Read the model definition and answer for the solid it produces. Units are mm, in the model's axes. A direction names the side the tool comes from. Give positions to 0.01 mm unless a question says otherwise; leave off trailing zeros. Write each loop counter-clockwise with the first axis right and the second up, starting at its lowest first coordinate (ties: lowest second). Pieces come first, ordered by that corner, then holes. Notation, with made-up numbers: (49.5, -16.5) -> (69.5, -16.5) arc R19 ccw to (69.5, -7.5) -> close; hole circle Ø11 at (26, -3.5). An arc over 180 degrees is marked (long way). Write item = value, one per line.
from build123d import *

# Parameters (mm, degrees)
F0_R          = 9.5
F1_DEPTH      = 42
F1_DEPTH_BACK = 59
F2_R          = 16
F3_DEPTH      = 2.5
F3_DEPTH_BACK = 2.5
F4_R          = 4


with BuildPart() as f1:
    # F0 (on Top) → F1 (new body, two sides)
    with BuildSketch(Plane.XY) as f1_sk:
        Circle(F0_R)
    extrude(amount=F1_DEPTH)
    extrude(f1_sk.sketch, amount=-F1_DEPTH_BACK)

    # F2 (on Top) → F3 (join, two sides)
    with BuildSketch(Plane.XY) as f3_sk:
        Circle(F2_R)
    extrude(amount=F3_DEPTH)
    extrude(f3_sk.sketch, amount=-F3_DEPTH_BACK)

    # F4
    f4_edges = [f1.edges().sort_by_distance(p)[0] for p in [
        (-9.5, 0, -2.5),
        (-9.5, 0, 2.5),
    ]]
    fillet(f4_edges, radius=F4_R)


solid = f1.part
(1) The part is cut by section C-C on z = -30. Determine the outline of the cut face in (x, y).
Checks:
outline = circle Ø19 at (0, 0)
(2) Given P1, Ø8, axis at y = -12, z = 20, coming from the -X side; P2, Ø5, axis at x = -11.5, y = -10, coming from the +Z side; P3, Ø10, axis at y = 11, z = 22, coming from the -X side, each flat-ended and moving along its own axis, determine where each tip first touches the part or whether it passes through.
Checks:
P1 = -5.12
P2 = 2.57
P3 = -7.37
(3) Consider L1, parallel to Z at x = 2, y = -13.5; L2, parallel to X at y = 3.5, z = 6.5; L3, parallel to X at y = 5.5, z = -12. Determine where each line is inside the solid, lowest interval first.
Checks:
L1 = -2.5 to 2.5
L2 = -8.83 to 8.83
L3 = -7.75 to 7.75
(4) A tool of negligible diameter and unlimited length cuts with its end or side. For faces 1 (the cylindrical face through (4.38, -8.43, -32.38)), 2 (the flat face through (0, 0, 42)), 3 (the flat face through (-7, -12, 2.5)), from which of +Z, -Z, +X, -X, +Y, -Y can it reach the whole face along a straight path? Write none if from no direction.
Checks:
face_1 = -Z
face_2 = +Z, +X, -X, +Y, -Y
face_3 = +Z
(5) The part is cut by section A-A on y = 0. Determine the outline of the cut face in (x, z), plus the area to 3 significant figures.
Checks:
outline = (-16, -2.5) -> (-13.5, -2.5) arc R4 cw to (-9.5, -6.5) -> (-9.5, -59) -> (9.5, -59) -> (9.5, -6.5) arc R4 cw to (13.5, -2.5) -> (16, -2.5) -> (16, 2.5) -> (13.5, 2.5) arc R4 cw to (9.5, 6.5) -> (9.5, 42) -> (-9.5, 42) -> (-9.5, 6.5) arc R4 cw to (-13.5, 2.5) -> (-16, 2.5) -> close
area = 2,000 mm²
